The listing builds one solid part. Answer for the finished solid, in the listing's coordinates (mm). Give positions to 0.01 mm unless a question says otherwise; leave off trailing zeros. Order: outer loops, then holes, each group sorted by start corner. A loop starts at its lowest first (then second) coordinate and runs counter-clockwise, first axis right, second up.
```python
from build123d import *

# Parameters (mm, degrees)
F0_W     = 90
F0_H     = 90
F1_DEPTH = 5
F2_D     = 6.5
F3_D     = 5.1054


with BuildPart() as f1:
    # F0 (on Top) → F1 (new body)
    with BuildSketch(Plane.XY):
        Rectangle(F0_W, F0_H)
    extrude(amount=F1_DEPTH)

    # F2 (through all)
    with Locations(Plane(origin=(0, 0, 0), x_dir=(1, 0, 0), z_dir=(0, 0, -1))):
        with Locations((-32.5, -32.5), (32.5, -32.5), (32.5, 32.5), (-32.5, 32.5)):
            Hole(F2_D / 2)

    # F3 (through all)
    with Locations(Plane(origin=(0, 0, 0), x_dir=(1, 0, 0), z_dir=(0, 0, -1))):
        with Locations((0, 0)):
            Hole(F3_D / 2)


solid = f1.part
```
1) Find section A-A (x = -32.5). Write down the section's boundary in (y, z).
Geometry says:
outline: (-45, 0) - (-35.75, 0) - (-35.75, 5) - (-45, 5) - close; (-29.25, 0) - (29.25, 0) - (29.25, 5) - (-29.25, 5) - close; (35.75, 0) - (45, 0) - (45, 5) - (35.75, 5) - close
2) Straight lines are drawn through the part: probe 1 along Y at (x, z) = (32.5, 1.8); probe 2 along Y at (x, z) = (34, 0.3). For each, find the intervals that lie inside material, in ascending order.
Geometry says:
probe 1: y = -45 to -35.75, -29.25 to 29.25, 35.75 to 45
probe 2: y = -45 to -35.38, -29.62 to 29.62, 35.38 to 45
3) For a pull along X with two mould halves and no side action, classify faces 1 (the flat face through (9, 1, 5)), 2 (the cylindrical face through (31, -29.617, 2.535)), 3 (the flat face through (-45, -1, 2)) as +X half, -X half, draft (parallel to the pull), parting line (faces both ways), or undercut.
Geometry says:
face 1: draft
face 2: undercut
face 3: -X half
4) Find section B-B (z = 4.1). Write down the section's boundary in (x, y).
Geometry says:
outline: (-45, -45) - (45, -45) - (45, 45) - (-45, 45) - close; hole circle Ø6.5 at (-32.5, -32.5); hole circle Ø6.5 at (-32.5, 32.5); hole circle Ø5.11 at (0, 0); hole circle Ø6.5 at (32.5, -32.5); hole circle Ø6.5 at (32.5, 32.5)
5) Find section C-C (x = 0). Write down the section's boundary in (y, z), then the cut area to 3 significant figures.
Geometry says:
outline: (-45, 0) - (-2.55, 0) - (-2.55, 5) - (-45, 5) - close; (2.55, 0) - (45, 0) - (45, 5) - (2.55, 5) - close
area: 424 mm2
